Answer from the drawing. Dimensions are ordinates in mm from the lowest x, y and z of the part. Coordinates: 2 decimals unless noted, no trailing zeros. Loops run counter-clockwise (first coordinate to the right, second up) from the corner with the lowest first, then second, coordinate; pieces in that order, holes last. Notation, with made-up numbers: (-18, 19.25) - (36, 19.25) arc R16 cw to (36, 48.25) - close; hole circle Ø3 at (81.25, 72). An arc over 180 degrees is marked (long way). One line per question, with ' | ' between items. Start each with the question number.
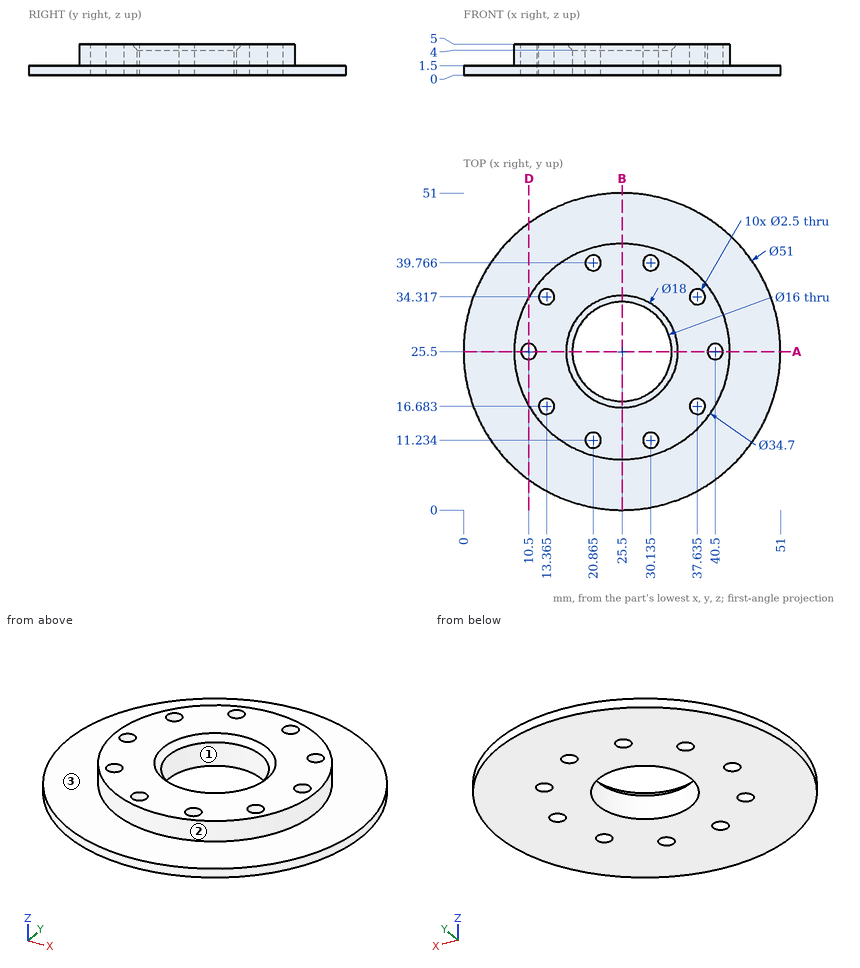
1) Given pin 1 Ø1.5 at (x, y) = (13.36, 16.68) entering from +Z; pin 2 Ø2 at (x, z) = (30, 1) entering from -Y; pin 3 Ø2 at (x, z) = (14, 0.5) entering from +Y; pin 4 Ø1.5 at (x, z) = (6, 2) entering from +Y, each flat-ended and moving along its own axis, determine where each tip first touches the part or whether it passes through.
2) The part is cut by section B-B on x = 25.5. Write down the section's boundary in (y, z).
3) The part is cut by section A-A on y = 25.5. Write down the section's boundary in (x, z).
4) The part is cut by section D-D on x = 10.5. Write down the section's boundary in (y, z), and give its area (3 significant figures).
5) Find the intervals of material crossed by line 1 along Y through (x, z) = (30, 4.35) (1 decimal); line 2 along X through (y, z) = (24, 2.2) (1 decimal); line 3 along Z through (x, y) = (42, 37.5), in increasing order. Write a range as from..to.
6) The mould has two halves that part along X. Classify the marked faces 1, 2 and 3: released by +X, released by -X, zero draft, split by the parting line, or undercut.
Answer below:
1) pin 1: through | pin 2: y = 0.24 | pin 3: y = 48.74 | pin 4: y = 42.57
2) outline: (0, 0) - (17.5, 0) - (17.5, 4) - (16.5, 5) - (8.15, 5) - (8.15, 1.5) - (0, 1.5) - close; (33.5, 0) - (51, 0) - (51, 1.5) - (42.85, 1.5) - (42.85, 5) - (34.5, 5) - (33.5, 4) - close
3) outline: (0, 0) - (9.25, 0) - (9.25, 5) - (8.15, 5) - (8.15, 1.5) - (0, 1.5) - close; (11.75, 0) - (17.5, 0) - (17.5, 4) - (16.5, 5) - (11.75, 5) - close; (33.5, 0) - (39.25, 0) - (39.25, 5) - (34.5, 5) - (33.5, 4) - close; (41.75, 0) - (51, 0) - (51, 1.5) - (42.85, 1.5) - (42.85, 5) - (41.75, 5) - close
4) outline: (4.88, 0) - (24.25, 0) - (24.25, 5) - (16.78, 5) - (16.78, 1.5) - (4.88, 1.5) - close; (26.75, 0) - (46.12, 0) - (46.12, 1.5) - (34.22, 1.5) - (34.22, 5) - (26.75, 5) - close | area: 110 mm2
5) line 1: 8.7..10, 12.5..18.5, 32.5..38.5, 41..42.3 | line 2: 8.2..17.6, 33.4..42.8 | line 3: 0..1.5
6) face 1: undercut | face 2: split by the parting line | face 3: zero draft
